Part print with two shaded views. Sizes in mm from the minimum x, y, z corner. A direction names the side the tool comes from. Give positions to 0.01 mm unless a question says otherwise; leave off trailing zeros. Loops run counter-clockwise (first coordinate to the right, second up) from the corner with the lowest first, then second, coordinate; pieces in that order, holes last. Notation, with made-up numbers: (54, 28.25) -> (72, 28.25) arc R18 cw to (72, 36.25) -> close; hole circle Ø7 at (84, 27.25). An arc over 180 degrees is marked (long way). One line per question, with ' | ' between items. Start each with the question number.
(1) Flat gauge pin, fed straight in: pin 1 Ø12 at (y, z) = (30.5, 52.5) entering from +X. Where does the tip first touch, or does it go through?
(2) 3-axis set-ups, long thin cutter, end or side, ignore diameter. For the marked faces 1 and 2: which of +Z, -Z, +X, -X, +Y, -Y reach the whole face in a straight line?
(3) Slice it at D-D, the plane z = 46. Write the cut outline in (x, y).
(4) Drill centre lines: L1, parallel to Z at x = 8.5, y = 5; L2, parallel to X at y = 38, z = 40; L3, parallel to Y at x = 5, z = 39 (1 decimal). Where is each one in solid material? Low to high. Write a range as from..to.
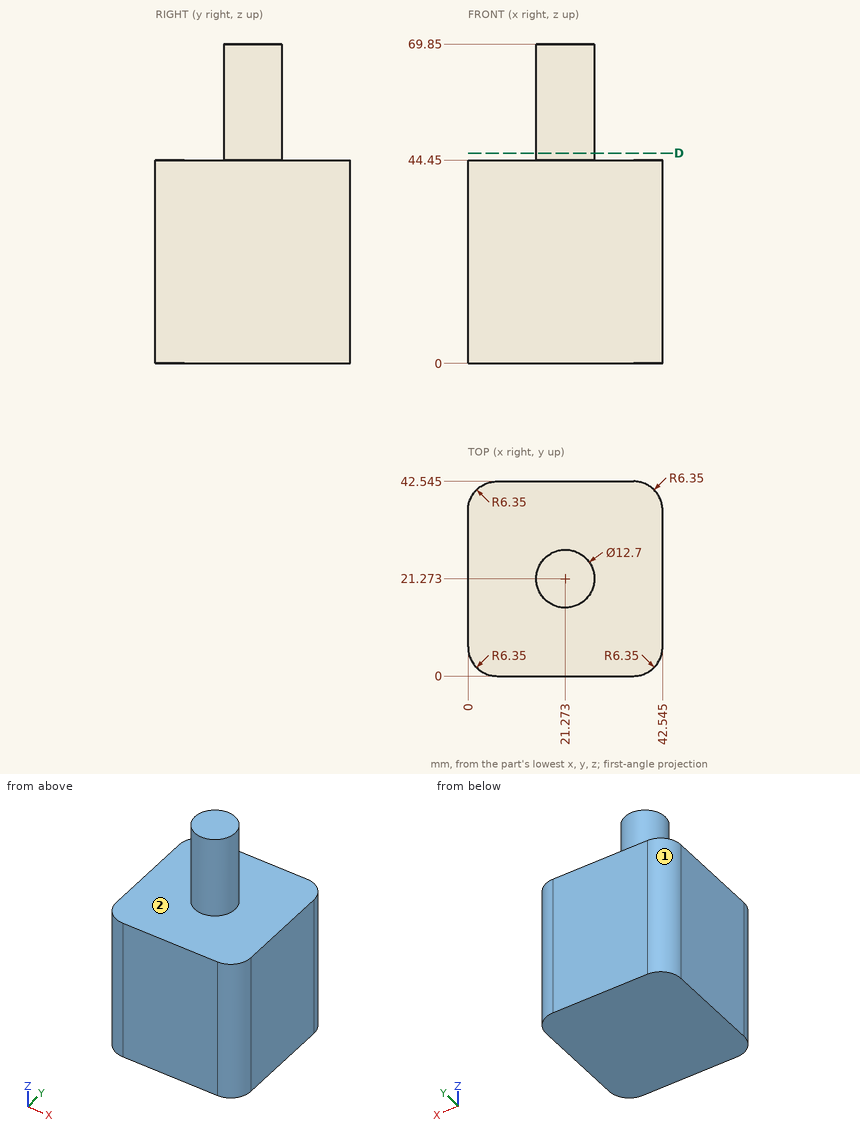
Final values:
1) pin 1: x = 26.74
2) face 1: +Z, -Z, -X, +Y | face 2: +Z
3) outline: circle Ø12.7 at (21.27, 21.27)
4) L1: 0..44.45 | L2: 0.26..42.28 | L3: 0.1..42.4
